Geometry check sheet. Reference: drawing and pictorial views, mm from the part's lowest x, y, z. A direction names the side the tool comes from. Coordinates: 2 decimals unless noted, no trailing zeros. Write each loop counter-clockwise with the first axis right and the second up, starting at its lowest first coordinate (ties: lowest second). Pieces come first, ordered by that corner, then holes. Notation, with made-up numbers: (88.5, 28) -> (132.5, 28) arc R24 cw to (132.5, 42) -> close; hole circle Ø3 at (-17, 7.25). An arc over 180 degrees is marked (long way). Answer in a Markdown table with one row per item.
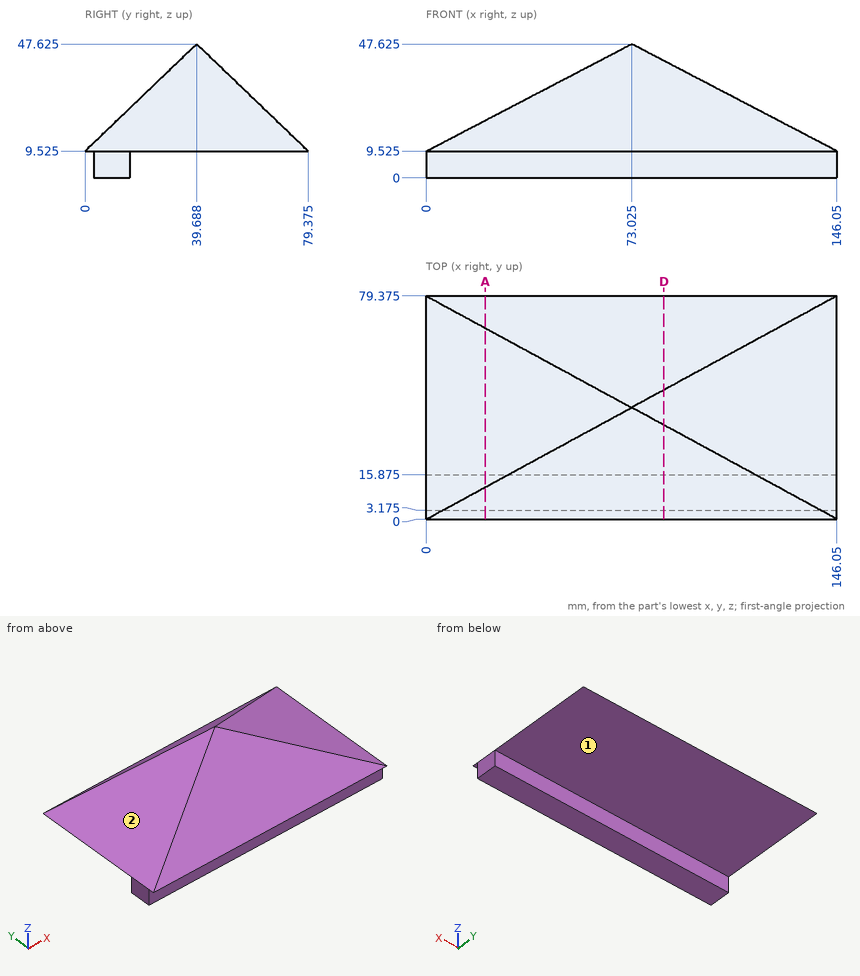
1. Depth check by flat-ended pin: P1, Ø6, axis at x = 81.5, z = 27, coming from the -Y side; P2, Ø12, axis at x = 46, y = 30, coming from the -Z side (1 decimal); P3, Ø1.5, axis at y = 60.5, z = 19.5, coming from the +X side. Enter the tip coordinate at first touch or a pass-through.
Geometry says:
| item | result |
|---|---|
| P1 | y = 15.08 |
| P2 | z = 9.5 |
| P3 | x = 128.37 |
2. Tool access check on the marked faces 1 and 2. Record the directions out of +Z, -Z, +X, -X, +Y, -Y that give a thin tool (end or side, any length) a straight path to the whole face; none if there is none.
Geometry says:
| item | result |
|---|---|
| face 1 | -Z, +X, -X, +Y |
| face 2 | +Z, -X, +Y, -Y |
3. Thickness scan on line 1 (Y direction, x = 139.5, z = 7) (1 decimal); line 2 (Z direction, x = 126.5, y = 71) (1 decimal); line 3 (Z direction, x = 103.5, y = 39) (1 decimal). Record the ranges inside material, lowest first. Write a range as from..to.
Geometry says:
| item | result |
|---|---|
| line 1 | 3.2..15.9 |
| line 2 | 9.5..17.6 |
| line 3 | 9.5..31.7 |
4. Section check D-D, the plane x = 84.5. Record the boundary of the cut face in (y, z) (1 decimal), plus the area to 3 significant figures.
Geometry says:
| item | result |
|---|---|
| outline | (0, 9.5) -> (3.2, 9.5) -> (3.2, 0) -> (15.9, 0) -> (15.9, 9.5) -> (79.4, 9.5) -> (45.9, 41.6) -> (33.5, 41.6) -> close |
| area | 1,600 mm^2 |
5. Section check A-A, the plane x = 21. Record the boundary of the cut face in (y, z) (1 decimal).
Geometry says:
| item | result |
|---|---|
| outline | (0, 9.5) -> (3.2, 9.5) -> (3.2, 0) -> (15.9, 0) -> (15.9, 9.5) -> (79.4, 9.5) -> (68, 20.5) -> (11.4, 20.5) -> close |
